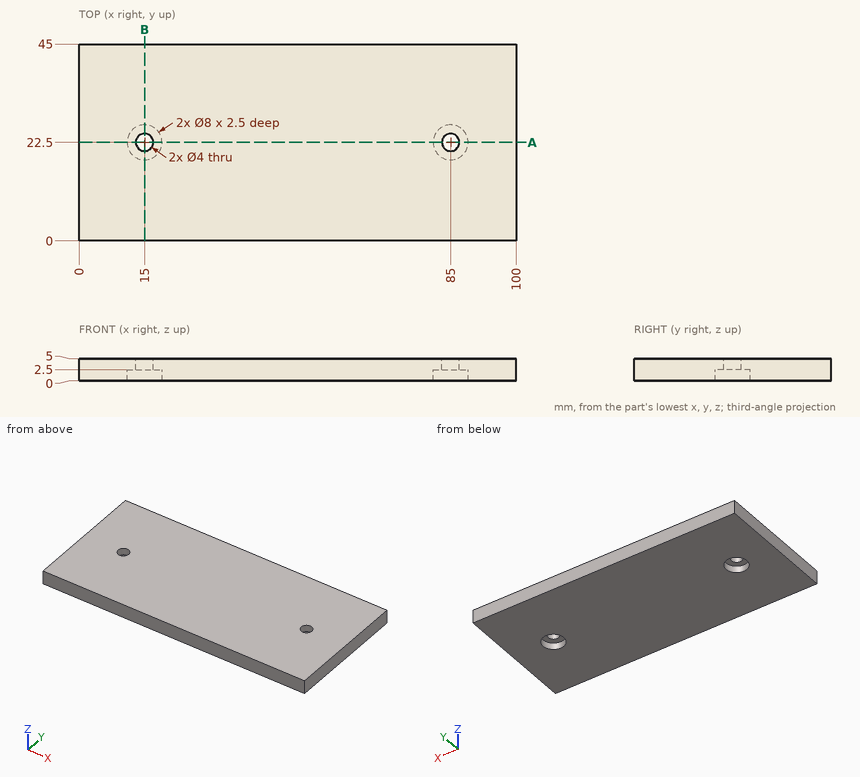
Answer from the drawing. Dimensions are ordinates in mm from the lowest x, y and z of the part. Round coordinates to 2 decimals unless told otherwise and drop trailing zeros. Loops run counter-clockwise (first coordinate to the right, second up) from the corner with the lowest first, then second, coordinate; pieces in that order, holes last.
(1) Find the intervals of material crossed by L1, parallel to X at y = 22.5, z = 1.65; L2, parallel to X at y = 22.5, z = 4.2; L3, parallel to Y at x = 85, z = 1.25, in increasing order.
Computed values:
L1: x = 0 to 11, 19 to 81, 89 to 100
L2: x = 0 to 13, 17 to 83, 87 to 100
L3: y = 0 to 18.5, 26.5 to 45
(2) This flat-tipped pin is pushed along its axis until it touches: P1, Ø5, axis at x = 85, y = 22.5, coming from the +Z side. Where does it stop, or does it pass through?
Computed values:
P1: stops at z = 5
(3) The part is cut by section B-B, the plane x = 15. Give the vertices of the cut face in (y, z), and give its area (3 significant figures).
Computed values:
outline: (0, 0) - (18.5, 0) - (18.5, 2.5) - (20.5, 2.5) - (20.5, 5) - (0, 5) - close; (24.5, 2.5) - (26.5, 2.5) - (26.5, 0) - (45, 0) - (45, 5) - (24.5, 5) - close
area: 195 mm2
(4) The part is cut by section A-A, the plane y = 22.5. Give the vertices of the cut face in (x, z), and give its area (3 significant figures).
Computed values:
outline: (0, 0) - (11, 0) - (11, 2.5) - (13, 2.5) - (13, 5) - (0, 5) - close; (17, 2.5) - (19, 2.5) - (19, 0) - (81, 0) - (81, 2.5) - (83, 2.5) - (83, 5) - (17, 5) - close; (87, 2.5) - (89, 2.5) - (89, 0) - (100, 0) - (100, 5) - (87, 5) - close
area: 440 mm2
